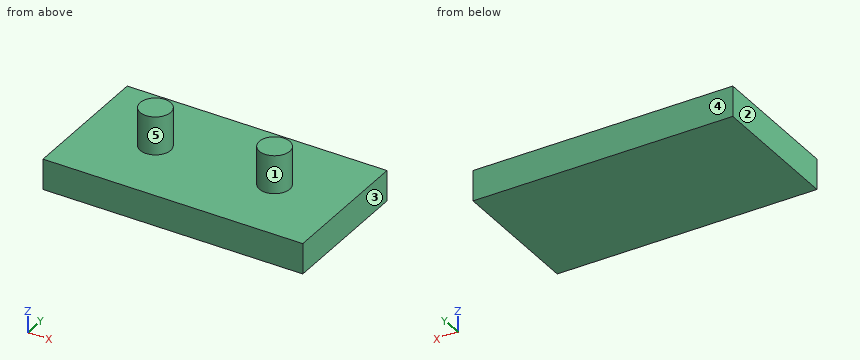
from build123d import *

# Parameters (mm, degrees)
F0_W     = 170
F0_H     = 90
F1_DEPTH = 20
F3_DEPTH = 25


with BuildPart() as f1:
    # F0 (on Top) → F1 (new body)
    with BuildSketch(Plane.XY):
        Rectangle(F0_W, F0_H)
    extrude(amount=F1_DEPTH)

    # F2 (on face) → F3 (join)
    with BuildSketch(Plane.XY.offset(20)):
        with BuildLine():
            Line((-49, 0), (-39, 0))
            Line((-39, 0), (-29, 0))
            ThreePointArc((-29, 0), (-39, 10), (-49, 0))
        make_face()
        with BuildLine():
            Line((-29, 0), (-39, 0))
            Line((-39, 0), (-49, 0))
            ThreePointArc((-49, 0), (-39, -10), (-29, 0))
        make_face()
        with BuildLine():
            ThreePointArc((49, 0), (39, 10), (29, 0))
            Line((29, 0), (39, 0))
            Line((39, 0), (49, 0))
        make_face()
        with BuildLine():
            Line((39, 0), (29, 0))
            ThreePointArc((29, 0), (39, -10), (49, 0))
            Line((49, 0), (39, 0))
        make_face()
    extrude(amount=F3_DEPTH)


solid = f1.part
Part model, mm, in its own coordinate system. Face numbers are marked on the shaded views. A direction names the side the tool comes from. Give positions to 0.01 mm unless a question says otherwise; leave off trailing zeros. Loops run counter-clockwise (first coordinate to the right, second up) from the corner with the lowest first, then second, coordinate; pieces in that order, holes last. Notation, with made-up numbers: M -10.75,55 L 36.25,55 A22 cw 36.25,77 Z; hole C 46.25,59 d4. An arc over 180 degrees is marked long. Put each result on its own line as item: value. Start each with the question number.
1) Saw through at A-A (y = 0). List the corners of the cut face in (x, z).
2) Saw through at C-C (z = 34). List the corners of the cut face in (x, y).
3) Saw through at B-B (x = -39). List the corners of the cut face in (y, z), then the cut area to 3 significant figures.
4) Pull direction X, two halves, no side cores. Call the marked faces 3, 4 and 5: +X half, -X half, draft (parallel to the pull), parting line (faces both ways), or undercut.
5) Probe probe 1 along Z at (x, y) = (-18.5, 15); probe 2 along X at (y, z) = (-3.5, 28.5). List the from-to ranges inside material, lowest first.
6) 3-axis set-ups, long thin cutter, end or side, ignore diameter. For the marked faces 1 and 2: which of +Z, -Z, +X, -X, +Y, -Y reach the whole face in a straight line?
7) Saw through at D-D (y = -17). List the corners of the cut face in (x, z).
8) Flat gauge pins, fed straight in: pin 1 (8 mm diameter, centred on x = -28, z = 36.5, fed in from +Y); pin 2 (1 mm diameter, centred on x = -56.5, z = 21.5, fed in from -Y); pin 3 (2 mm diameter, centred on x = 53, y = -21.5, fed in from +Z); pin 4 (5 mm diameter, centred on x = 27.5, z = 38.5, fed in from +Y). Where does each tip first touch, or does it go through?
Numbers:
1. outline: M -85,0 L 85,0 L 85,20 L 49,20 L 49,45 L 29,45 L 29,20 L -29,20 L -29,45 L -49,45 L -49,20 L -85,20 Z
2. outline: C -39,0 d20; C 39,0 d20
3. outline: M -45,0 L 45,0 L 45,20 L 10,20 L 10,45 L -10,45 L -10,20 L -45,20 Z
3. area: 2,300 mm^2
4. face 3: +X half
4. face 4: draft
4. face 5: undercut
5. probe 1: 0 to 20
5. probe 2: -48.37 to -29.63, 29.63 to 48.37
6. face 1: +Z
6. face 2: +Z, -Z, -X, +Y, -Y
7. outline: M -85,0 L 85,0 L 85,20 L -85,20 Z
8. pin 1: y = 7.14
8. pin 2: through
8. pin 3: z = 20
8. pin 4: y = 4.36
